```python
from build123d import *

# Parameters (mm, degrees)
SKETCH_262_W         = 80
SKETCH_262_H         = 130
EXTRUDE_1_DEPTH      = 14
SKETCH_1_W           = 77
SKETCH_1_H           = 127
CUT_EXTRUDE_1_DEPTH  = 12.5
CUT_EXTRUDE_2_DEPTH  = 2
SKETCH_10_W          = 8
SKETCH_10_H          = 12
EXTRUDE_2_DEPTH      = 6.9
SKETCH_11_W          = 12.6
SKETCH_11_H          = 1
EXTRUDE_3_DEPTH      = 12
SKETCH_13_R          = 3.5
EXTRUDE_4_DEPTH      = 28
CUT_EXTRUDE_9_DEPTH  = 1.5
CUT_EXTRUDE_START    = -1.5
CUT_EXTRUDE_10_DEPTH = 1.5
CUT_EXTRUDE_11_DEPTH = 1.5
CUT_EXTRUDE_12_DEPTH = 1.5
SKETCH_15_R          = 1.5
CUT_EXTRUDE_14_DEPTH = 19.5
SKETCH_16_W          = 30
SKETCH_16_H          = 2
EXTRUDE_5_DEPTH      = 2
SKETCH_17_W          = 1
SKETCH_17_H          = 14
EXTRUDE_6_DEPTH      = 12


with BuildPart() as part:
    # Sketch 262 → Бобышка-Вытянуть1 (new body)
    with BuildSketch(Plane(origin=(0, 0, 0), x_dir=(1, 0, 0), z_dir=(0, 1, 0))):
        Rectangle(SKETCH_262_W, SKETCH_262_H)
    extrude(amount=EXTRUDE_1_DEPTH)

    # Эскиз1 → Вырез-Вытянуть1 (cut)
    with BuildSketch(Plane(origin=(0, 14, 0), x_dir=(1, 0, 0), z_dir=(0, 1, 0))):
        Rectangle(SKETCH_1_W, SKETCH_1_H)
    extrude(amount=-CUT_EXTRUDE_1_DEPTH, mode=Mode.SUBTRACT)

    # Эскиз2 → Вырез-Вытянуть2 (cut)
    with BuildSketch(Plane.XY.offset(-63.5)):
        with BuildLine():
            Line((-9, 18.3), (-9.5, 18.3))
            ThreePointArc((-9.5, 18.3), (-12.5, 15.3), (-9.5, 12.3))
            Line((-9.5, 12.3), (-9, 12.3))
            Line((-9, 12.3), (-9, 6.3))
            Line((-9, 6.3), (9, 6.3))
            Line((9, 6.3), (9, 12.3))
            Line((9, 12.3), (9.5, 12.3))
            ThreePointArc((9.5, 12.3), (12.5, 15.3), (9.5, 18.3))
            Line((9.5, 18.3), (9, 18.3))
            Line((9, 18.3), (9, 24.3))
            Line((9, 24.3), (-9, 24.3))
            Line((-9, 24.3), (-9, 18.3))
        make_face()
    extrude(amount=-CUT_EXTRUDE_2_DEPTH, mode=Mode.SUBTRACT)

    # Эскиз10 → Бобышка-Вытянуть2 (add)
    with BuildSketch(Plane(origin=(0, 1.5, 0), x_dir=(1, 0, 0), z_dir=(0, 1, 0))):
        with Locations((-29.9, 44)):
            Rectangle(SKETCH_10_W, SKETCH_10_H)
        with Locations((29.9, 44)):
            Rectangle(SKETCH_10_W, SKETCH_10_H)
        with Locations((-29.9, -54)):
            Rectangle(SKETCH_10_W, SKETCH_10_H)
        with Locations((29.9, -54)):
            Rectangle(SKETCH_10_W, SKETCH_10_H)
    extrude(amount=EXTRUDE_2_DEPTH)

    # Эскиз11 → Бобышка-Вытянуть3 (add)
    with BuildSketch(Plane(origin=(0, 1.5, 0), x_dir=(1, 0, 0), z_dir=(0, 1, 0))):
        with Locations((-32.2, 50.5)):
            Rectangle(SKETCH_11_W, SKETCH_11_H)
        with Locations((32.2, 50.5)):
            Rectangle(SKETCH_11_W, SKETCH_11_H)
        with Locations((-32.2, 37.5)):
            Rectangle(SKETCH_11_W, SKETCH_11_H)
        with Locations((32.2, 37.5)):
            Rectangle(SKETCH_11_W, SKETCH_11_H)
        with Locations((32.2, -47.5)):
            Rectangle(SKETCH_11_W, SKETCH_11_H)
        with Locations((32.2, -60.5)):
            Rectangle(SKETCH_11_W, SKETCH_11_H)
        with Locations((-32.2, -47.5)):
            Rectangle(SKETCH_11_W, SKETCH_11_H)
        with Locations((-32.2, -60.5)):
            Rectangle(SKETCH_11_W, SKETCH_11_H)
    extrude(amount=EXTRUDE_3_DEPTH)

    # Эскиз13 → Бобышка-Вытянуть4 (add)
    with BuildSketch(Plane(origin=(0, 1.5, 0), x_dir=(1, 0, 0), z_dir=(0, 1, 0))):
        with Locations(Location((-34.5, 33, 0), (0, 0, 270))):
            Circle(SKETCH_13_R)
        with Locations(Location((34.5, 33, 0), (0, 0, 270))):
            Circle(SKETCH_13_R)
        with Locations(Location((-34.5, -43, 0), (0, 0, 270))):
            Circle(SKETCH_13_R)
        with Locations(Location((34.5, -43, 0), (0, 0, 270))):
            Circle(SKETCH_13_R)
    extrude(amount=EXTRUDE_4_DEPTH)

    # Эскиз5 → Вырез-Вытянуть9 (cut)
    with BuildSketch(Plane.ZY.offset(40)):
        with BuildLine():
            Line((57.199546833, 20.146147769), (57.196157558, 19.944779244))
            ThreePointArc((57.196157558, 19.944779244), (54, 8), (50.803842442, 19.944779244))
            Line((50.803842442, 19.944779244), (50.800453167, 20.146147769))
            ThreePointArc((50.800453167, 20.146147769), (54, 23.4), (57.199546833, 20.146147769))
        make_face()
    extrude(amount=-CUT_EXTRUDE_9_DEPTH, mode=Mode.SUBTRACT)

    # Эскиз6 → Вырез-Вытянуть10 (cut)
    with BuildSketch(Plane(origin=(40, 0, 0), x_dir=(0, 0, -1), z_dir=(1, 0, 0)).offset(CUT_EXTRUDE_START)):
        with BuildLine():
            Line((-50.8, 20.2), (-50.8, 19.942562584))
            ThreePointArc((-50.8, 19.942562584), (-54, 8), (-57.2, 19.942562584))
            Line((-57.2, 19.942562584), (-57.2, 20.2))
            ThreePointArc((-57.2, 20.2), (-54, 23.4), (-50.8, 20.2))
        make_face()
    extrude(amount=CUT_EXTRUDE_10_DEPTH, mode=Mode.SUBTRACT)

    # Эскиз3 → Вырез-Вытянуть11 (cut)
    with BuildSketch(Plane.ZY.offset(40)):
        with BuildLine():
            Line((-40.8, 20.2), (-40.8, 19.942562584))
            ThreePointArc((-40.8, 19.942562584), (-44, 8), (-47.2, 19.942562584))
            Line((-47.2, 19.942562584), (-47.2, 20.2))
            ThreePointArc((-47.2, 20.2), (-44, 23.4), (-40.8, 20.2))
        make_face()
    extrude(amount=-CUT_EXTRUDE_11_DEPTH, mode=Mode.SUBTRACT)

    # Эскиз9 → Вырез-Вытянуть12 (cut)
    with BuildSketch(Plane(origin=(40, 0, 0), x_dir=(0, 0, -1), z_dir=(1, 0, 0)).offset(CUT_EXTRUDE_START)):
        with BuildLine():
            Line((47.2, 20.2), (47.2, 19.942562584))
            ThreePointArc((47.2, 19.942562584), (44, 8), (40.8, 19.942562584))
            Line((40.8, 19.942562584), (40.8, 20.2))
            ThreePointArc((40.8, 20.2), (44, 23.4), (47.2, 20.2))
        make_face()
    extrude(amount=CUT_EXTRUDE_12_DEPTH, mode=Mode.SUBTRACT)

    # Эскиз15 → Вырез-Вытянуть14 (cut)
    with BuildSketch(Plane(origin=(0, 29.5, 0), x_dir=(1, 0, 0), z_dir=(0, 1, 0))):
        with Locations(Location((-34.5, 33, 0), (0, 0, 270))):
            Circle(SKETCH_15_R)
        with Locations(Location((34.5, 33, 0), (0, 0, 270))):
            Circle(SKETCH_15_R)
        with Locations(Location((34.5, -43, 0), (0, 0, 270))):
            Circle(SKETCH_15_R)
        with Locations(Location((-34.5, -43, 0), (0, 0, 270))):
            Circle(SKETCH_15_R)
    extrude(amount=-CUT_EXTRUDE_14_DEPTH, mode=Mode.SUBTRACT)

    # Эскиз16 → Бобышка-Вытянуть5 (add)
    with BuildSketch(Plane(origin=(0, 1.5, 0), x_dir=(1, 0, 0), z_dir=(0, 1, 0))):
        with Locations((0, 62.5)):
            Rectangle(SKETCH_16_W, SKETCH_16_H)
        with Locations((0, 58)):
            Rectangle(SKETCH_16_W, SKETCH_16_H)
    extrude(amount=EXTRUDE_5_DEPTH)

    # Эскиз17 → Бобышка-Вытянуть6 (add)
    with BuildSketch(Plane(origin=(0, 1.5, 0), x_dir=(1, 0, 0), z_dir=(0, 1, 0))):
        with Locations((-13, 44)):
            Rectangle(SKETCH_17_W, SKETCH_17_H)
        with Locations((13, 44)):
            Rectangle(SKETCH_17_W, SKETCH_17_H)
        with Locations((-13, -54)):
            Rectangle(SKETCH_17_W, SKETCH_17_H)
        with Locations((13, -54)):
            Rectangle(SKETCH_17_W, SKETCH_17_H)
    extrude(amount=EXTRUDE_6_DEPTH)


solid = part.part
```
Geometry: final body of the model. Coordinates: model frame, mm. A direction names the side the tool comes from. Give positions to 0.01 mm unless a question says otherwise; leave off trailing zeros. Order: outer loops, then holes, each group sorted by start corner. A loop starts at its lowest first (then second) coordinate and runs counter-clockwise, first axis right, second up. Notation, with made-up numbers: (38.5, 53) -> (72.5, 53) arc R20 ccw to (72.5, 81) -> close; hole circle Ø9 at (26, 12). An arc over 180 degrees is marked (long way). Write each question's results on one line, items separated by ' | '. Start each with the question number.
1) First-contact query: pin 1 (5 mm diameter, centred on x = 36.5, z = 51.5, fed in from +Y); pin 2 (0.8 mm diameter, centred on x = 39.5, z = -14.5, fed in from +Y); pin 3 (1.5 mm diameter, centred on x = -34.5, z = -33.5, fed in from +Y); pin 4 (12 mm diameter, centred on x = 16.5, y = 21.5, fed in from +Z). Flat tips, straight axial feed; report the tip coordinate or a pass-through.
2) Set-up query: faces 4 (the cylindrical face through (-39, 8, -44)), 5 (the cylindrical face through (39, 8, 54)), 6 (the flat face through (-36, 1.5, 54)). Return all of +Z, -Z, +X, -X, +Y, -Y with unobstructed straight access to the full face (end or side cutting, diameter ignored); none if empty.
3) Section A-A (y = 18). Return loops of the section in (x, z), then the cut area to 3 significant figures.
4) Draft query along Z for faces 1 (the flat face through (40, 7, 1)), 2 (the flat face through (-1, 7, 65)), 3 (the flat face through (-34, 10, -33)). Return one class per face: pulls with the +Z half, pulls with the -Z half, needs draft (parallel to the pull), parting line crosses it, or undercut.
5) Section C-C (z = 43). Return loops of the section in (x, y), then the cut area to 4 significant figures.
6) Line query: line 1 (X direction, y = 24.25, z = 43); line 2 (X direction, y = 13.25, z = 52.5); line 3 (X direction, y = 13.25, z = 37). Output: solid intervals per line, ascending. Write a range as from..to.
7) Section B-B (x = 29). Return loops of the section in (y, z), then the cut area to 3 significant figures.
8) Section D-D (y = 4.75). Count the separate pieces of the cut face and the enclosed holes in it, then the cut area to 3 significant figures.
Calculated:
1) pin 1: y = 9.4 | pin 2: y = 14 | pin 3: y = 10 | pin 4: through
2) face 4: -X, +Y | face 5: +X, +Y | face 6: +Y
3) outline: circle Ø7 at (-34.5, -33); circle Ø7 at (-34.5, 43); circle Ø7 at (34.5, -33); circle Ø7 at (34.5, 43); hole circle Ø3 at (-34.5, -33); hole circle Ø3 at (-34.5, 43); hole circle Ø3 at (34.5, -33); hole circle Ø3 at (34.5, 43) | area: 126 mm2
4) face 1: needs draft | face 2: pulls with the +Z half | face 3: undercut
5) outline: (-40, 0) -> (40, 0) -> (40, 14) -> (38.5, 14) -> (38.5, 1.5) -> (38, 1.5) -> (38, 29.5) -> (36, 29.5) -> (36, 10) -> (33, 10) -> (33, 29.5) -> (31, 29.5) -> (31, 1.5) -> (-31, 1.5) -> (-31, 29.5) -> (-33, 29.5) -> (-33, 10) -> (-36, 10) -> (-36, 29.5) -> (-38, 29.5) -> (-38, 1.5) -> (-38.5, 1.5) -> (-38.5, 14) -> (-40, 14) -> close | area: 432.5 mm2
6) line 1: -38..-36, -33..-31, 31..33, 36..38 | line 2: -13.5..-12.5, 12.5..13.5 | line 3: -40..-38.5, 38.5..40
7) outline: (0, -65) -> (14, -65) -> (14, -63.5) -> (1.5, -63.5) -> (1.5, -51) -> (13.5, -51) -> (13.5, -50) -> (8.4, -50) -> (8.4, -38) -> (13.5, -38) -> (13.5, -37) -> (1.5, -37) -> (1.5, 47) -> (13.5, 47) -> (13.5, 48) -> (8.4, 48) -> (8.4, 60) -> (13.5, 60) -> (13.5, 61) -> (1.5, 61) -> (1.5, 63.5) -> (14, 63.5) -> (14, 65) -> (0, 65) -> close | area: 446 mm2
8) separate pieces: 9 | enclosed holes: 5 | area: 1,320 mm2
